Could you check a few things on this drawing? It's one solid part, dimensions in mm from its lowest x, y, z. Coordinates: 2 decimals unless noted, no trailing zeros. Loops run counter-clockwise (first coordinate to the right, second up) from the corner with the lowest first, then second, coordinate; pieces in that order, holes last. Notation, with made-up numbers: M 71.5,34.5 L 111.5,34.5 A26 ccw 111.5,61.5 Z; hole C 64.25,42 d10. An arc over 180 degrees is marked long. Use one line per item in the form item = value. Start each with the question number.
(1) Please list where these lines run through material, in increasing order: L1, parallel to Z at x = 18.75, y = 301.5; L2, parallel to Y at x = 11.5, z = 173; L3, parallel to Y at x = 18.25, z = 163.
(2) Imagine slicing it at A-A, the plane x = 13.5. Please give me the cut outline in (y, z).
(3) Imagine slicing it at B-B, the plane y = 103.5. Please give me the cut outline in (x, z).
(4) Imagine slicing it at C-C, the plane z = 190. Please give me the cut outline in (x, y).
(5) Will these pins go through, and if not, where does the flat tip stop? P1, Ø5, axis at x = 14, y = 130, coming from the -Z side; P2, Ø5, axis at x = 22, z = 104, coming from the -Y side; P3, Ø3, axis at y = 323.5, z = 166.5, coming from the -X side.
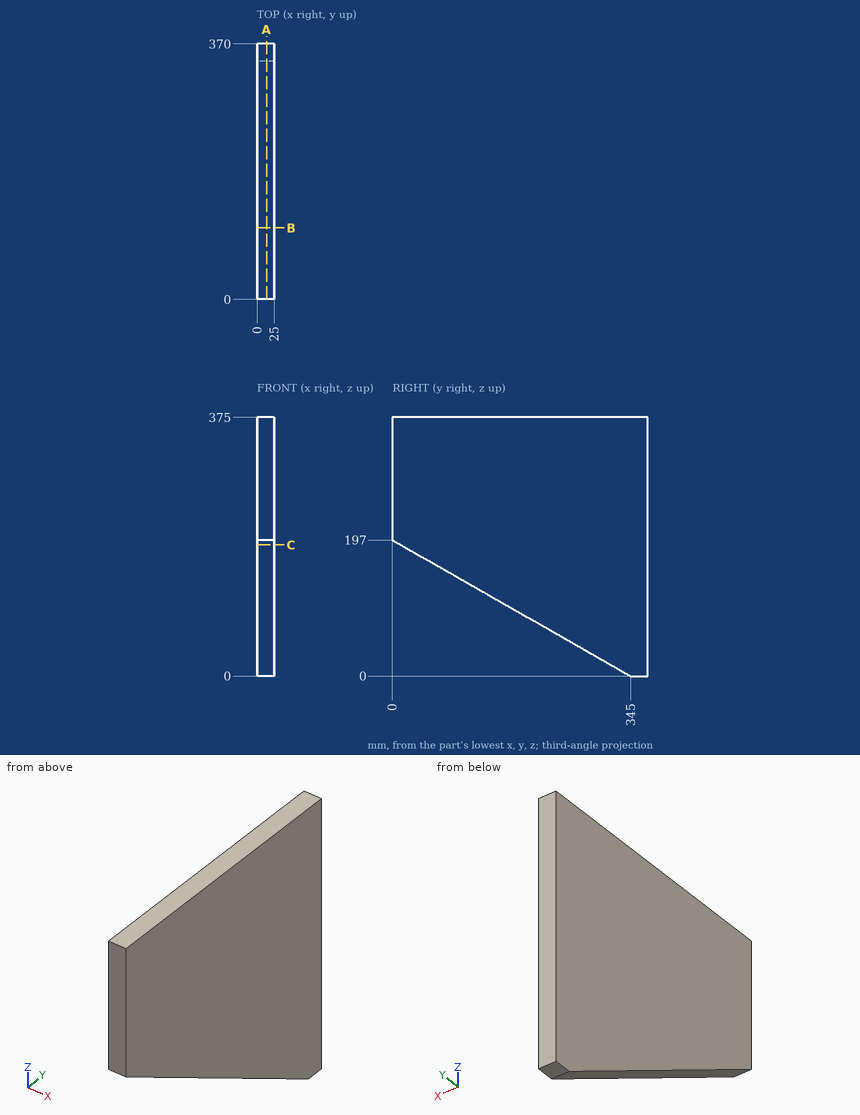
Answer:
q1.L1 = 24.84 to 375
q1.L2 = 42.03 to 370
q1.L3 = 59.54 to 370
q2.outline = M 0,197 L 345,0 L 370,0 L 370,375 L 0,375 Z
q3.outline = M 0,137.9 L 25,137.9 L 25,375 L 0,375 Z
q4.outline = M 0,12.26 L 25,12.26 L 25,370 L 0,370 Z
q5.P1 = 121.34
q5.P2 = 158.49
q5.P3 = 0
